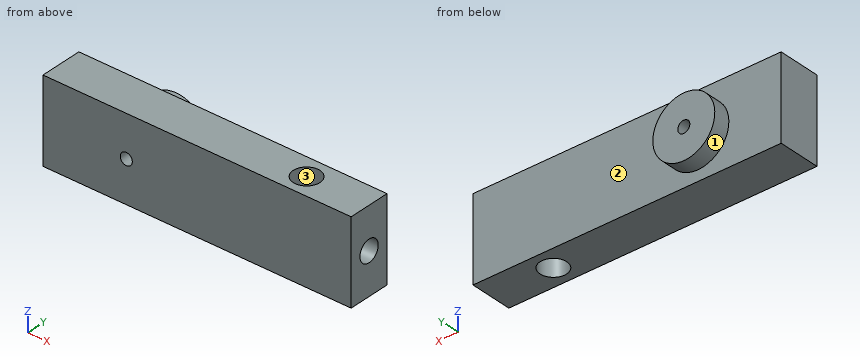
from build123d import *

# Parameters (mm, degrees)
SKETCH_1_W               = 15
SKETCH_1_H               = 10
EXTRUDE_1_DEPTH          = 5.1
SKETCH_2_R               = 1.6
CUT_EXTRUDE_1_DEPTH      = 14.500370365
SKETCH_3_R               = 1.3
CUT_EXTRUDE_2_DEPTH      = 3.8
CUT_EXTRUDE_3_REACH      = 15.283
CUT_EXTRUDE_3_END_RADIUS = 1.6
SKETCH_4_R               = 0.575
SKETCH_5_W               = 10
SKETCH_5_H               = 5.1
EXTRUDE_2_DEPTH          = 22
SKETCH_6_R               = 3.72
EXTRUDE_3_DEPTH          = 2
SKETCH_7_R               = 0.725
CUT_EXTRUDE_4_DEPTH      = 31.751585341


with BuildPart() as part:
    # 草图1 → 凸台-拉伸1 (new body)
    with BuildSketch(Plane(origin=(0, 0, 0), x_dir=(1, 0, 0), z_dir=(0, 1, 0))):
        Rectangle(SKETCH_1_W, SKETCH_1_H)
    extrude(amount=EXTRUDE_1_DEPTH)

    # 草图2 → 切除-拉伸1 (cut, through all)
    with BuildSketch(Plane.XY.offset(5)):
        with Locations((0, 2.55)):
            Circle(SKETCH_2_R)
    extrude(amount=-CUT_EXTRUDE_1_DEPTH, mode=Mode.SUBTRACT)

    # 草图3 → 切除-拉伸2 (cut)
    with BuildSketch(Plane(origin=(7.5, 0, 0), x_dir=(0, 0, -1), z_dir=(1, 0, 0))):
        with Locations((0, 2.55)):
            Circle(SKETCH_3_R)
    extrude(amount=-CUT_EXTRUDE_2_DEPTH, mode=Mode.SUBTRACT)

    # 切除-拉伸3: up to this cylinder (the profile starts outside it)
    cut_extrude_3_end = Plane(origin=(0, 2.55, 0), z_dir=(0, 0, 1)) * Cylinder(CUT_EXTRUDE_3_END_RADIUS, 34.766, mode=Mode.PRIVATE)
    # 草图4 → 切除-拉伸3 (cut, up to the surface)
    with BuildSketch(Plane(origin=(3.7, 0, 0), x_dir=(0, 0, -1), z_dir=(1, 0, 0)), mode=Mode.PRIVATE) as cut_extrude_3_sk1:
        with Locations((0, 2.55)):
            Circle(SKETCH_4_R)
    cut_extrude_3_tool1 = extrude(cut_extrude_3_sk1.sketch, amount=-CUT_EXTRUDE_3_REACH, mode=Mode.PRIVATE) - cut_extrude_3_end
    add(cut_extrude_3_tool1.solids().sort_by_distance((3.7, 2.55, 0))[0], mode=Mode.SUBTRACT)

    # 草图5 → 凸台-拉伸2 (add)
    with BuildSketch(Plane.ZY.offset(7.5)):
        with Locations((0, 2.55)):
            Rectangle(SKETCH_5_W, SKETCH_5_H)
    extrude(amount=EXTRUDE_2_DEPTH)

    # 草图6 → 凸台-拉伸3 (add)
    with BuildSketch(Plane(origin=(0, 5.1, 0), x_dir=(1, 0, 0), z_dir=(0, 1, 0))):
        with Locations(Location((-19.5, 0, 0), (0, 0, 270))):
            Circle(SKETCH_6_R)
    extrude(amount=EXTRUDE_3_DEPTH)

    # 草图7 → 切除-拉伸4 (cut, through all)
    with BuildSketch(Plane(origin=(0, 7.1, 0), x_dir=(1, 0, 0), z_dir=(0, 1, 0))):
        with Locations(Location((-19.5, 0, 0), (0, 0, 270))):
            Circle(SKETCH_7_R)
    extrude(amount=-CUT_EXTRUDE_4_DEPTH, mode=Mode.SUBTRACT)


solid = part.part
Geometry check sheet. Reference: the model listing, model coordinates, mm. Face numbers are marked on the shaded views. Give positions to 0.01 mm unless a question says otherwise; leave off trailing zeros. Order: outer loops, then holes, each group sorted by start corner. A loop starts at its lowest first (then second) coordinate and runs counter-clockwise, first axis right, second up. Notation, with made-up numbers: (-10, 20) - (6, 20) arc R29 ccw to (6, 54) - close; hole circle Ø2 at (-15.5, 41). An arc over 180 degrees is marked (long way). Use one line per item in the form item = value.
1) Sectioned sample at C-C (z = 0). Record the boundary of the cut face in (x, y) (3 decimals).
Working result:
outline = (-29.5, 0) - (-20.225, 0) - (-20.225, 7.1) - (-23.22, 7.1) - (-23.22, 5.1) - (-29.5, 5.1) - close; (-18.775, 0) - (7.5, 0) - (7.5, 1.25) - (3.7, 1.25) - (3.7, 1.975) - (1.493, 1.975) arc R1.6 cw (long way) to (1.493, 3.125) - (3.7, 3.125) - (3.7, 3.85) - (7.5, 3.85) - (7.5, 5.1) - (-15.78, 5.1) - (-15.78, 7.1) - (-18.775, 7.1) - close
2) Sectioned sample at B-B (x = 0). Record the boundary of the cut face in (y, z).
Working result:
outline = (0, -5) - (0.95, -5) - (0.95, 5) - (0, 5) - close; (4.15, -5) - (5.1, -5) - (5.1, 5) - (4.15, 5) - close
3) Material ranges on probe 1 along Y at (x, z) = (5.8, 0); probe 2 along X at (y, z) = (2.5, -4); probe 3 along Y at (x, z) = (0, 0.25), recorded low to high. Write a range as from..to.
Working result:
probe_1 = 0..1.25, 3.85..5.1
probe_2 = -29.5..-1.6, 1.6..7.5
probe_3 = 0..0.95, 4.15..5.1
4) Sectioned sample at A-A (y = 2.55). Record the boundary of the cut face in (x, z) (3 decimals).
Working result:
outline = (-29.5, -5) - (-1.6, -5) - (-1.6, 5) - (-29.5, 5) - close; (1.6, -5) - (7.5, -5) - (7.5, -1.3) - (3.7, -1.3) - (3.7, -0.575) - (1.6, -0.575) - close; (1.6, 0.575) - (3.7, 0.575) - (3.7, 1.3) - (7.5, 1.3) - (7.5, 5) - (1.6, 5) - close; hole circle Ø1.45 at (-19.5, 0)
5) Sectioned sample at D-D (z = 4.25). Record the boundary of the cut face in (x, y), and give its area (3 significant figures).
Working result:
outline = (-29.5, 0) - (7.5, 0) - (7.5, 5.1) - (-29.5, 5.1) - close; hole circle Ø3.2 at (0, 2.55)
area = 181 mm^2
6) Draft check along X on the marked faces 1, 2 and 3. Enter one of: released by +X, released by -X, zero draft, split by the parting line, or undercut.
Working result:
face_1 = split by the parting line
face_2 = zero draft
face_3 = undercut
7) Depth check by flat-ended pin: pin 1 Ø1.3 at (y, z) = (2.55, 0) entering from +X; pin 2 Ø1 at (x, z) = (-0.5, -0.5) entering from +Y. Enter the tip coordinate at first touch or a pass-through.
Working result:
pin_1 = 3.7
pin_2 = 5.1
